Design review of the part built by this model. Coordinates are the model's own, in mm. Face numbers are marked on the shaded views. A direction names the side the tool comes from. Coordinates: 2 decimals unless noted, no trailing zeros. Loops run counter-clockwise (first coordinate to the right, second up) from the corner with the lowest first, then second, coordinate; pieces in that order, holes last. Notation, with made-up numbers: (50, 76.5) -> (82, 76.5) arc R31 ccw to (82, 109.5) -> close; hole circle Ø7 at (70, 12). An arc over 180 degrees is marked (long way). Use CSV: the item, a comma, the result in double quotes.
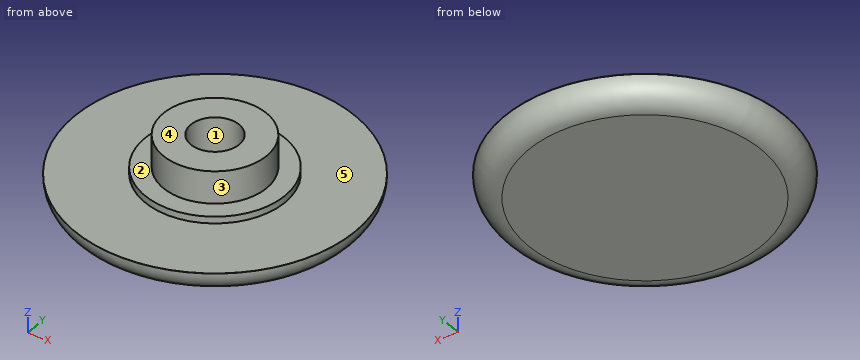
```python
from build123d import *

# Parameters (mm, degrees)
F0_R     = 11.0236
F1_DEPTH = 1.905
F2_R     = 5.50545
F3_DEPTH = 0.5334
F4_R     = 4.064
F5_DEPTH = 2.54
F6_R     = 1.905
F7_DEPTH = 3.0734
F8_R     = 1.8542


with BuildPart() as f1:
    # F0 (on Top) → F1 (new body)
    with BuildSketch(Plane.XY):
        Circle(F0_R)
    extrude(amount=F1_DEPTH)

    # F2 (on face) → F3 (join)
    with BuildSketch(Plane.XY.offset(1.905)):
        Circle(F2_R)
    extrude(amount=F3_DEPTH)

    # F4 (on face) → F5 (join)
    with BuildSketch(Plane.XY.offset(2.4384)):
        Circle(F4_R)
    extrude(amount=F5_DEPTH)

    # F6 (on face) → F7 (cut, through all)
    with BuildSketch(Plane.XY.offset(4.9784)):
        Circle(F6_R)
    extrude(amount=-F7_DEPTH, mode=Mode.SUBTRACT)

    # F8
    f8_edges = [f1.edges().sort_by_distance(p)[0] for p in [
        (-11.0236, 0, 0),
    ]]
    fillet(f8_edges, radius=F8_R)


solid = f1.part
```
Item 1: Add section B-B (z = 3). Give the boundary of the cut face in (x, y) (3 decimals), then the cut area to 3 significant figures.
Checked values:
outline,"circle Ø8.128 at (0, 0); hole circle Ø3.81 at (0, 0)"
area,"40.5 mm^2"
Item 2: To check wall thickness, follow line 1 along Y through (x, z) = (0, 4.3) (3 decimals); line 2 along Z through (x, y) = (7.5, 2) (3 decimals); line 3 along Y through (x, z) = (3.5, 1.05). State the ranges of each line that lie inside material, in increasing order.
Checked values:
line 1,"-4.064 to -1.905, 1.905 to 4.064"
line 2,"0 to 1.905"
line 3,"-10.26 to 10.26"
Item 3: Machinability: for the marked faces 4 and 5, which of the approach directions +Z, -Z, +X, -X, +Y, -Y give a long, thin tool a straight path to every point of the face, cutting with its end or side? Answer none if there is none.
Checked values:
face 4,"+Z, +X, -X, +Y, -Y"
face 5,"+Z"
Item 4: Add section A-A (y = 0). Give the boundary of the cut face in (x, z) (3 decimals), then the cut area to 3 significant figures.
Checked values:
outline,"(-11.024, 1.854) arc R1.854 ccw to (-9.169, 0) -> (9.169, 0) arc R1.854 ccw to (11.024, 1.854) -> (11.024, 1.905) -> (5.505, 1.905) -> (5.505, 2.438) -> (4.064, 2.438) -> (4.064, 4.978) -> (1.905, 4.978) -> (1.905, 1.905) -> (-1.905, 1.905) -> (-1.905, 4.978) -> (-4.064, 4.978) -> (-4.064, 2.438) -> (-5.505, 2.438) -> (-5.505, 1.905) -> (-11.024, 1.905) -> close"
area,"55.3 mm^2"
Item 5: Draft analysis for pull direction Y (two halves, no side actions). For the marked faces 1, 2 and 3, state which applies: pulls with the +Y half, pulls with the -Y half, needs draft (parallel to the pull), parting line crosses it, or undercut.
Checked values:
face 1,"undercut"
face 2,"needs draft"
face 3,"parting line crosses it"
Item 6: Clearance check with flat-ended pins moving along their axes: pin 1 (2 mm diameter, centred on y = -4, z = 0.5, fed in from -X); pin 2 (1.1 mm diameter, centred on x = 0, y = 0.5, fed in from +Z) (3 decimals); pin 3 (2 mm diameter, centred on y = 0, z = 4.5, fed in from -X). State where each tip first meets the part, or that it passes through.
Checked values:
pin 1,"x = -10.4"
pin 2,"z = 1.905"
pin 3,"x = -4.06"
